Build history of the part. All positions in model axes, mm. A direction names the side the tool comes from. Round coordinates to 2 decimals unless told otherwise and drop trailing zeros. Loops run counter-clockwise (first coordinate to the right, second up) from the corner with the lowest first, then second, coordinate; pieces in that order, holes last. Notation, with made-up numbers: (8, -1) -> (19, -1) arc R24 cw to (19, 21) -> close; hole circle Ø3 at (-6.5, 5.5). An arc over 180 degrees is marked (long way). Put each result on its own line as item: value. Start each with the question number.
Item 1: Cut at C-C, the plane x = -4.5. List the corners of the cut face in (y, z) (1 decimal).
Item 2: Pull direction Z, two halves, no side cores. Call faces 1 (the flat face through (6, 6, -6)), 2 (the cylindrical face through (0.159, 3.874, -0.86)): +Z half, -Z half, draft (parallel to the pull), parting line (faces both ways), or undercut.
Item 3: Flat gauge pins, fed straight in: pin 1 Ø2.5 at (y, z) = (-1, 1) entering from +X; pin 2 Ø6 at (y, z) = (-3, -1) entering from -X; pin 3 Ø10.5 at (y, z) = (0, 0) entering from +X. Where does each tip first touch, or does it go through?
Item 4: Cut at A-A, the plane y = 0. List the corners of the cut face in (x, z).
Item 5: Cut at D-D, the plane x = 2.5. List the corners of the cut face in (y, z) (1 decimal).
Item 6: Tool access for faces 3 (the cylindrical face through (-3.36, 7.75, -1.72)), 4 (the flat face through (-6, 6, 6)), 5 (the cylindrical face through (3.44, 7.75, -1.72)): list every direction of +Z, -Z, +X, -X, +Y, -Y with a clear straight run to the whole face (end or side of a thin tool).
Item 7: Drill centre lines: probe 1 along X at (y, z) = (3.5, -0.5); probe 2 along X at (y, z) = (4.5, 0.25); probe 3 along Z at (x, y) = (1, 2.5). Where is each one in solid material? Low to high. Write a range as [from, to].
```python
from build123d import *


# Not quite as in the source:
# - a feature names something its author has since deleted; it is built from what else it names


with BuildPart() as f1:
    # F0 (on Front) → F1 (revolve)
    with BuildSketch(Plane.XZ):
        with BuildLine():
            Line((6, 7.9375), (6, 13.5))
            ThreePointArc((6, 13.5), (0, 10.5), (-6, 13.5))
            Line((-6, 13.5), (-6, 7.9375))
            Line((-6, 7.9375), (-0.8, 7.9375))
            Line((-0.8, 7.9375), (-0.8, 0))
            Line((-0.8, 0), (-0.5, 0))
            Line((-0.5, 0), (-0.5, 3.96875))
            Line((-0.5, 3.96875), (0.8, 3.96875))
            Line((0.8, 3.96875), (0.8, 7.9375))
            Line((0.8, 7.9375), (6, 7.9375))
        make_face()
    revolve(axis=Axis((-0.4498892081, 0, 0), (1, 0, 0)))


solid = f1.part
```
Reply:
1. outline: circle Ø24 at (0, 0); hole circle Ø15.9 at (0, 0)
2. face 1: draft
2. face 2: undercut
3. pin 1: stops at x = -0.5
3. pin 2: stops at x = -0.8
3. pin 3: stops at x = 0.8
4. outline: (-6, -13.5) arc R7.5 cw to (6, -13.5) -> (6, -7.94) -> (0.8, -7.94) -> (0.8, -3.97) -> (-0.5, -3.97) -> (-0.5, 3.97) -> (0.8, 3.97) -> (0.8, 7.94) -> (6, 7.94) -> (6, 13.5) arc R7.5 cw to (-6, 13.5) -> (-6, 7.94) -> (-0.8, 7.94) -> (-0.8, -7.94) -> (-6, -7.94) -> close
5. outline: circle Ø21.9 at (0, 0); hole circle Ø15.9 at (0, 0)
6. face 3: -X
6. face 4: +Z, -Z, -X, +Y, -Y
6. face 5: +X
7. probe 1: x = [-0.8, -0.5]
7. probe 2: x = [-0.8, 0.8]
7. probe 3: z = [-10.27, -7.53], [7.53, 10.27]
